For this review, take the finished solid that the model builds, in its own axes (mm). Coordinates: 2 decimals unless noted, no trailing zeros. Order: outer loops, then holes, each group sorted by start corner. A loop starts at its lowest first (then second) coordinate and runs counter-clockwise, first axis right, second up. Notation, with made-up numbers: (49, -5.5) -> (62, -5.5) arc R19 ccw to (62, 18.5) -> close; hole circle Ø10 at (76, 57). An arc over 180 degrees is marked (long way). Return JSON: item names as keys, results as strings. Group by question number.
Item 1: Insertion check: pin 1 (3 mm diameter, centred on y = 59.5, z = 6, fed in from +X); pin 2 (4 mm diameter, centred on x = -1, z = 5.5, fed in from +Y); pin 3 (6 mm diameter, centred on x = -4.5, z = 2.5, fed in from +Y). Each pin has a flat end and moves straight along its axis. Give the tip position at first contact, or say it passes through.
Item 2: Take a section at C-C (z = 4.75). Count the separate pieces of the cut face and the enclosed holes in it, then the cut area to 3 significant figures.
Item 3: Draft analysis for pull direction X (two halves, no side actions). For faces 1 (the conical face through (67.48, -48.48, 2.85)), 2 (the flat face through (-2, 2, 10)), state which applies: +X half, -X half, draft (parallel to the pull), parting line (faces both ways), or undercut.
Item 4: For line 1 along Y through (x, z) = (55, 4.5); line 2 along Y through (x, z) = (-63, 2.25); line 3 along Y through (x, z) = (-9, 2.5), list the stretches that pass through material, from the lowest coordinate up.
Item 5: Take a section at A-A (x = 0). Write out the cut boundary in (y, z), then the cut area to 3 significant figures.
```python
from build123d import *

# Parameters (mm, degrees)
F1_R     = 125
F1_R_2   = 15
F2_DEPTH = 10
F3_R     = 8
F4_SIZE  = 3


with BuildPart() as f2:
    # F1 (on face) → F2 (new body)
    with BuildSketch(Plane.XY):
        Circle(F1_R)
        with Locations((-53.033009, -53.033009)):
            Circle(F1_R_2, mode=Mode.SUBTRACT)
        with Locations((0, -75)):
            Circle(F1_R_2, mode=Mode.SUBTRACT)
        with Locations((53.033009, -53.033009)):
            Circle(F1_R_2, mode=Mode.SUBTRACT)
        with Locations((-75, 0)):
            Circle(F1_R_2, mode=Mode.SUBTRACT)
        with Locations((-53.033009, 53.033009)):
            Circle(F1_R_2, mode=Mode.SUBTRACT)
        with Locations((53.033009, 53.033009)):
            Circle(F1_R_2, mode=Mode.SUBTRACT)
        with Locations((75, 0)):
            Circle(F1_R_2, mode=Mode.SUBTRACT)
        with Locations((0, 75)):
            Circle(F1_R_2, mode=Mode.SUBTRACT)
    extrude(amount=F2_DEPTH)

    # F3
    f3_edges = [f2.edges().sort_by_distance(p)[0] for p in [
        (-125, 0, 10),
    ]]
    fillet(f3_edges, radius=F3_R)

    # F4
    f4_edges = [f2.edges().sort_by_distance(p)[0] for p in [
        (-68.033009, -53.033009, 10),
        (-90, 0, 10),
        (-68.033009, 53.033009, 10),
        (-15, 75, 10),
        (38.033009, 53.033009, 10),
        (60, 0, 10),
        (38.033009, -53.033009, 10),
        (-15, -75, 10),
        (38.033009, -53.033009, 0),
        (60, 0, 0),
        (38.033009, 53.033009, 0),
        (-15, 75, 0),
        (-68.033009, 53.033009, 0),
        (-90, 0, 0),
        (-68.033009, -53.033009, 0),
        (-15, -75, 0),
    ]]
    chamfer(f4_edges, length=F4_SIZE)


solid = f2.part
```
Findings below:
{
 "1": {"pin 1": "stops at x = 109.87", "pin 2": "stops at y = 124.85", "pin 3": "stops at y = 124.99"},
 "2": {"separate pieces": "1", "enclosed holes": "8", "area": "43,100 mm2"},
 "3": {"face 1": "undercut", "face 2": "draft"},
 "4": {"line 1": "y = -111.8 to -67.9, -38.16 to 38.16, 67.9 to 111.8", "line 2": "y = -107.96 to -65.23, -40.84 to -10.2, 10.2 to 40.84, 65.23 to 107.96", "line 3": "y = -124.66 to -87.62, -62.38 to 62.38, 87.62 to 124.66"},
 "5": {"outline": "(-125, 0) -> (-93, 0) -> (-90, 3) -> (-90, 7) -> (-93, 10) -> (-117, 10) arc R8 ccw to (-125, 2) -> close; (-60, 3) -> (-57, 0) -> (57, 0) -> (60, 3) -> (60, 7) -> (57, 10) -> (-57, 10) -> (-60, 7) -> close; (90, 3) -> (93, 0) -> (125, 0) -> (125, 2) arc R8 ccw to (117, 10) -> (93, 10) -> (90, 7) -> close", "area": "1,840 mm2"}
}
